```python
from build123d import *

# Parameters (mm, degrees)
SKETCH1_W           = 92
SKETCH1_H           = 56
BOSS_EXTRUDE1_DEPTH = 12
SKETCH8_W           = 92
SKETCH8_H           = 2
BOSS_EXTRUDE3_DEPTH = 12
CUT_EXTRUDE1_REACH  = 58.214
SKETCH2_R           = 10.5
CUT_EXTRUDE5_REACH  = 58.214
FILLET2_R           = 12
CUT_EXTRUDE7_REACH  = 58.214
SKETCH12_R          = 10.5


with BuildPart() as part:
    # Sketch1 → Boss-Extrude1 (new body)
    with BuildSketch(Plane(origin=(0, 0, 0), x_dir=(1, 0, 0), z_dir=(0, 1, 0))):
        Rectangle(SKETCH1_W, SKETCH1_H)
    extrude(amount=BOSS_EXTRUDE1_DEPTH)

    # Sketch8 → Boss-Extrude3 (add)
    with BuildSketch(Plane(origin=(0, 12, 0), x_dir=(1, 0, 0), z_dir=(0, 1, 0))):
        with Locations((0, 29)):
            Rectangle(SKETCH8_W, SKETCH8_H)
    extrude(amount=-BOSS_EXTRUDE3_DEPTH)

    # Sketch2 → Cut-Extrude1 (cut, up to next)
    with BuildSketch(Plane(origin=(0, 12, 0), x_dir=(1, 0, 0), z_dir=(0, 1, 0)), mode=Mode.PRIVATE) as cut_extrude1_sk1:
        with Locations(Location((-25, -1.5, 0), (0, 0, 270))):
            Circle(SKETCH2_R)
    cut_extrude1_tool1 = extrude(cut_extrude1_sk1.sketch, amount=-CUT_EXTRUDE1_REACH, mode=Mode.PRIVATE) & part.part
    # Sketch2 → Cut-Extrude1 (cut, up to next)
    with BuildSketch(Plane(origin=(0, 12, 0), x_dir=(1, 0, 0), z_dir=(0, 1, 0)), mode=Mode.PRIVATE) as cut_extrude1_sk2:
        with Locations(Location((25, -1.5, 0), (0, 0, 270))):
            Circle(SKETCH2_R)
    cut_extrude1_tool2 = extrude(cut_extrude1_sk2.sketch, amount=-CUT_EXTRUDE1_REACH, mode=Mode.PRIVATE) & part.part
    add(cut_extrude1_tool1.solids().sort_by_distance((-25, 12, 1.5))[0], mode=Mode.SUBTRACT)
    add(cut_extrude1_tool2.solids().sort_by_distance((25, 12, 1.5))[0], mode=Mode.SUBTRACT)

    # Sketch10 → Cut-Extrude5 (cut, up to next)
    with BuildSketch(Plane(origin=(0, 12, 0), x_dir=(1, 0, 0), z_dir=(0, 1, 0)), mode=Mode.PRIVATE) as cut_extrude5_sk1:
        with BuildLine():
            Line((-46, 5.057438524), (-46, 30))
            Line((-46, 30), (-16, 30))
            Line((-16, 30), (-35.667304108, 17.740806196))
            ThreePointArc((-35.667304108, 17.740806196), (-42.056420822, 12.395269294), (-46, 5.057438524))
        make_face()
    cut_extrude5_tool1 = extrude(cut_extrude5_sk1.sketch, amount=-CUT_EXTRUDE5_REACH, mode=Mode.PRIVATE) & part.part
    # Sketch10 → Cut-Extrude5 (cut, up to next)
    with BuildSketch(Plane(origin=(0, 12, 0), x_dir=(1, 0, 0), z_dir=(0, 1, 0)), mode=Mode.PRIVATE) as cut_extrude5_sk2:
        with BuildLine():
            Line((46, 5.057438524), (46, 30))
            Line((46, 30), (16, 30))
            Line((16, 30), (36.615382461, 17.183760068))
            ThreePointArc((36.615382461, 17.183760068), (42.39835371, 11.964668142), (46, 5.057438524))
        make_face()
    cut_extrude5_tool2 = extrude(cut_extrude5_sk2.sketch, amount=-CUT_EXTRUDE5_REACH, mode=Mode.PRIVATE) & part.part
    add(cut_extrude5_tool1.solids().sort_by_distance((-36.403407, 12, -23.114901))[0], mode=Mode.SUBTRACT)
    add(cut_extrude5_tool2.solids().sort_by_distance((36.411287, 12, -23.11647))[0], mode=Mode.SUBTRACT)

    # Fillet2
    fillet2_edges = [part.edges().sort_by_distance(p)[0] for p in [
        (-16, 6, -30),
        (16, 6, -30),
    ]]
    fillet(fillet2_edges, radius=FILLET2_R)

    # Sketch12 → Cut-Extrude7 (cut, up to next)
    with BuildSketch(Plane.XZ, mode=Mode.PRIVATE) as cut_extrude7_sk1:
        with Locations(Location((0, -16.5, 0), (0, 0, 270))):
            Circle(SKETCH12_R)
    cut_extrude7_tool1 = extrude(cut_extrude7_sk1.sketch, amount=-CUT_EXTRUDE7_REACH, mode=Mode.PRIVATE) & part.part
    add(cut_extrude7_tool1.solids().sort_by_distance((0, 0, -16.5))[0], mode=Mode.SUBTRACT)


solid = part.part
```
Read the model definition and answer for the solid it produces. Units are mm, in the model's axes. Coordinates: 2 decimals unless noted, no trailing zeros. Write each loop counter-clockwise with the first axis right and the second up, starting at its lowest first coordinate (ties: lowest second). Pieces come first, ordered by that corner, then holes. Notation, with made-up numbers: (42, 80.25) - (86, 80.25) arc R18 cw to (86, 89.25) - close; hole circle Ø3 at (34.25, -3.5). An arc over 180 degrees is marked (long way). Answer as a JSON object with one key per item and string values. Group by question number.
1. A cutting plane is placed at C-C (y = 5.5). Determine the outline of the cut face in (x, z), plus the area to 3 significant figures.
2. A cutting plane is placed at A-A (x = 0). Determine the outline of the cut face in (y, z), plus the area to 3 significant figures.
3. Consider L1, parallel to X at y = 7.75, z = 1.5; L2, parallel to X at y = 2.25, z = 3; L3, parallel to X at y = 9, z = -25. Determine where each line is inside the solid, lowest interval first. Write a range as [from, to].
4. The mould has two halves that part along X. Classify faces 1 (the cylindrical face through (42.33, 6.08, -12.05)), 2 (the flat face through (-1, 0, 5)), 3 (the cylindrical face through (3.2, 5.9, -26.5)): +X half, -X half, draft (parallel to the pull), parting line (faces both ways), or undercut.
5. A cutting plane is placed at B-B (z = 1.5). Determine the outline of the cut face in (x, y), plus the area to 3 significant figures.
6. A cutting plane is placed at D-D (x = 20.5). Determine the outline of the cut face in (y, z).
7. Each of these flat-tipped pins is pushed along its axis until it touches: P1, Ø1, axis at y = 1.5, z = -7, coming from the -X side; P2, Ø1.5, axis at y = 2, z = -8, coming from the -X side. Where does it stop, or does it pass through?
Worked out:
{
 "1": {"outline": "(-46, -5.06) arc R22 ccw to (-35.67, -17.74) - (-18.91, -28.18) arc R12 ccw to (-12.57, -30) - (12.57, -30) arc R12 ccw to (18.91, -28.19) - (36.62, -17.18) arc R22 ccw to (46, -5.06) - (46, 28) - (-46, 28) - close; hole circle Ø21 at (-25, 1.5); hole circle Ø21 at (0, -16.5); hole circle Ø21 at (25, 1.5)", "area": "3,700 mm²"},
 "2": {"outline": "(0, -30) - (12, -30) - (12, -27) - (0, -27) - close; (0, -6) - (12, -6) - (12, 28) - (0, 28) - close", "area": "444 mm²"},
 "3": {"L1": "x = [-46, -35.5], [-14.5, 14.5], [35.5, 46]", "L2": "x = [-46, -35.39], [-14.61, 14.61], [35.39, 46]", "L3": "x = [-24.02, -6.16], [6.16, 24.04]"},
 "4": {"face 1": "+X half", "face 2": "draft", "face 3": "undercut"},
 "5": {"outline": "(-46, 0) - (-35.5, 0) - (-35.5, 12) - (-46, 12) - close; (-14.5, 0) - (14.5, 0) - (14.5, 12) - (-14.5, 12) - close; (35.5, 0) - (46, 0) - (46, 12) - (35.5, 12) - close", "area": "600 mm²"},
 "6": {"outline": "(0, -27.2) - (12, -27.2) - (12, -7.99) - (0, -7.99) - close; (0, 10.99) - (12, 10.99) - (12, 28) - (0, 28) - close"},
 "7": {"P1": "stops at x = -45.49", "P2": "stops at x = -45.19"}
}
